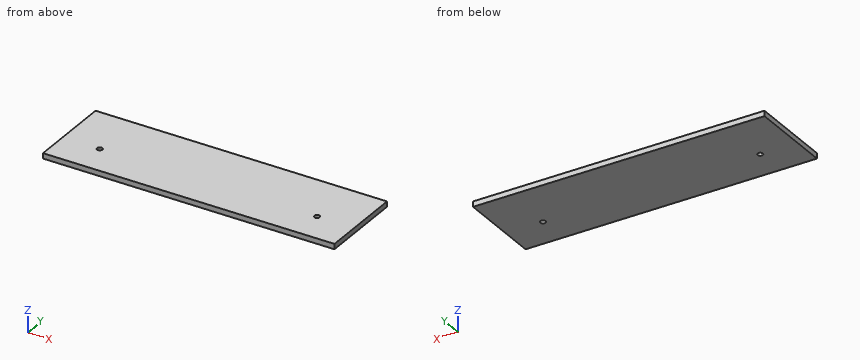
```python
from build123d import *

# Parameters (mm, degrees)
SKETCH1_W           = 55
SKETCH1_H           = 20
BOSS_EXTRUDE1_DEPTH = 1
SKETCH2_R           = 0.5
CUT_EXTRUDE1_DEPTH  = 59.532042507
SKETCH4_W           = 55
SKETCH4_H           = 4.024392025
CUT_EXTRUDE3_DEPTH  = 5


with BuildPart() as part:
    # Sketch1 → Boss-Extrude1 (new body)
    with BuildSketch(Plane.XY):
        with Locations((27.5, -10)):
            Rectangle(SKETCH1_W, SKETCH1_H)
    extrude(amount=BOSS_EXTRUDE1_DEPTH)

    # Sketch2 → Cut-Extrude1 (cut, through all)
    with BuildSketch(Plane.XY.offset(1)):
        with Locations((7, -10)):
            Circle(SKETCH2_R)
    cut_extrude1 = extrude(amount=-CUT_EXTRUDE1_DEPTH, mode=Mode.SUBTRACT)

    # Mirror2: Cut-Extrude1 across plane
    add(cut_extrude1.mirror(Plane.ZY.offset(-27.5)), mode=Mode.SUBTRACT)

    # Sketch4 → Cut-Extrude3 (cut)
    with BuildSketch(Plane.XY.offset(1)):
        with Locations((27.5, -17.987803988)):
            Rectangle(SKETCH4_W, SKETCH4_H)
    extrude(amount=-CUT_EXTRUDE3_DEPTH, mode=Mode.SUBTRACT)


solid = part.part
```
The listing builds one solid part. Answer for the finished solid, in the listing's coordinates (mm). Give positions to 0.01 mm unless a question says otherwise; leave off trailing zeros. Loops run counter-clockwise (first coordinate to the right, second up) from the corner with the lowest first, then second, coordinate; pieces in that order, holes last. Notation, with made-up numbers: (11.5, -18) - (60.5, -18) arc R30 ccw to (60.5, 14) - close; hole circle Ø3 at (-1, -24). An arc over 180 degrees is marked (long way). Answer as CSV lines item,"result". Start each with the question number.
Item 1: A cutting plane is placed at B-B on y = -10. Determine the outline of the cut face in (x, z), then the cut area to 3 significant figures.
Item 2: A cutting plane is placed at A-A on x = 48. Determine the outline of the cut face in (y, z), then the cut area to 3 significant figures.
Item 3: Find the intervals of material crossed by line 1 (Y direction, x = 48, z = 0.75); line 2 (X direction, y = -10.25, z = 0.6), in increasing order. Write a range as from..to.
Item 4: This flat-tipped pin is pushed along its axis until it touches: pin 1 (5 mm diameter, centred on x = 10.5, y = -4, fed in from -Z). Where does it stop, or does it pass through?
Found:
1,outline,"(0, 0) - (6.5, 0) - (6.5, 1) - (0, 1) - close; (7.5, 0) - (47.5, 0) - (47.5, 1) - (7.5, 1) - close; (48.5, 0) - (55, 0) - (55, 1) - (48.5, 1) - close"
1,area,"53.0 mm^2"
2,outline,"(-15.98, 0) - (-10.5, 0) - (-10.5, 1) - (-15.98, 1) - close; (-9.5, 0) - (0, 0) - (0, 1) - (-9.5, 1) - close"
2,area,"15.0 mm^2"
3,line 1,"y = -15.98..-10.5, -9.5..0"
3,line 2,"x = 0..6.57, 7.43..47.57, 48.43..55"
4,pin 1,"stops at z = 0"
